The listing builds one solid part. Answer for the finished solid, in the listing's coordinates (mm). Give positions to 0.01 mm unless a question says otherwise; leave off trailing zeros. Order: outer loops, then holes, each group sorted by start corner. A loop starts at its lowest first (then second) coordinate and runs counter-clockwise, first axis right, second up.
```python
from build123d import *

# Parameters (mm, degrees)
SKETCH1_W           = 1155
SKETCH1_H           = 80
BOSS_EXTRUDE1_DEPTH = 12
SKETCH2_R           = 9
CUT_EXTRUDE1_DEPTH  = 580.007987855
LPATTERN1_COUNT     = 4
LPATTERN1_PITCH     = 366
SKETCH3_W           = 60
SKETCH3_H           = 98
SKETCH3_R           = 10
BOSS_EXTRUDE2_DEPTH = 12
SKETCH4_W           = 60
SKETCH4_H           = 12
BOSS_EXTRUDE3_DEPTH = 52.5
SKETCH6_W           = 60
SKETCH6_H           = 110
SKETCH6_R           = 10
BOSS_EXTRUDE4_DEPTH = 12
SKETCH7_W           = 60
SKETCH7_H           = 98
CUT_EXTRUDE2_DEPTH  = 12


with BuildPart() as part:
    # Sketch1 → Boss-Extrude1 (new body)
    with BuildSketch(Plane(origin=(0, 0, 0), x_dir=(1, 0, 0), z_dir=(0, 1, 0))):
        Rectangle(SKETCH1_W, SKETCH1_H)
    extrude(amount=BOSS_EXTRUDE1_DEPTH)

    # Sketch2 → Cut-Extrude1 (cut, symmetric)
    with BuildSketch(Plane(origin=(0, 12, 0), x_dir=(1, 0, 0), z_dir=(0, 1, 0))):
        with Locations(Location((-549, 0, 0), (0, 0, 270))):
            Circle(SKETCH2_R)
    cut_extrude1 = extrude(amount=CUT_EXTRUDE1_DEPTH, both=True, mode=Mode.SUBTRACT)

    # LPattern1: Cut-Extrude1 ×4
    with Locations(*[(i * LPATTERN1_PITCH, 0, 0) for i in range(1, LPATTERN1_COUNT)]):
        add(cut_extrude1, mode=Mode.SUBTRACT)

    # Sketch3 → Boss-Extrude2 (add)
    with BuildSketch(Plane(origin=(0, 12, 0), x_dir=(1, 0, 0), z_dir=(0, 1, 0))):
        with Locations((-427.5, -89)):
            Rectangle(SKETCH3_W, SKETCH3_H)
        with Locations(Location((-427.5, -108, 0), (0, 0, 270))):
            Circle(SKETCH3_R, mode=Mode.SUBTRACT)
    extrude(amount=-BOSS_EXTRUDE2_DEPTH)

    # Sketch4 → Boss-Extrude3 (add)
    with BuildSketch(Plane(origin=(0, 0, 0), x_dir=(-1, 0, 0), z_dir=(0, -1, 0))):
        with Locations((427.5, -34)):
            Rectangle(SKETCH4_W, SKETCH4_H)
    extrude(amount=BOSS_EXTRUDE3_DEPTH)

    # Sketch6 → Boss-Extrude4 (add)
    with BuildSketch(Plane.XZ.offset(52.5)):
        with Locations((-427.5, 83)):
            Rectangle(SKETCH6_W, SKETCH6_H)
        with Locations(Location((-427.5, 108, 0), (0, 0, 90))):
            Circle(SKETCH6_R, mode=Mode.SUBTRACT)
    extrude(amount=BOSS_EXTRUDE4_DEPTH)

    # Sketch7 → Cut-Extrude2 (cut)
    with BuildSketch(Plane(origin=(0, 12, 0), x_dir=(1, 0, 0), z_dir=(0, 1, 0))):
        with Locations((-427.5, -89)):
            Rectangle(SKETCH7_W, SKETCH7_H)
    extrude(amount=-CUT_EXTRUDE2_DEPTH, mode=Mode.SUBTRACT)


solid = part.part
```
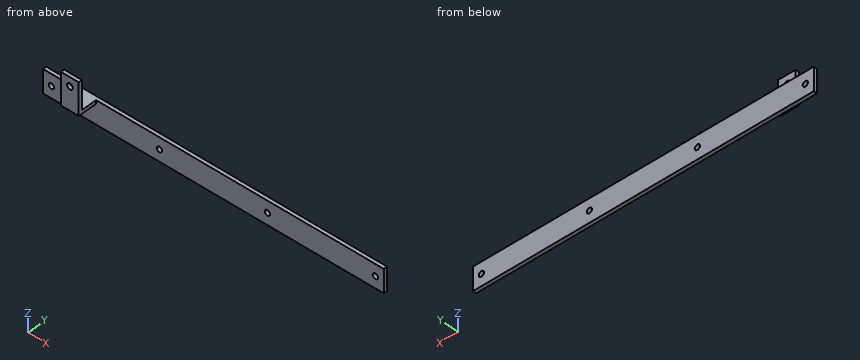
1) Find section C-C (y = -25). Write down the section's boundary in (x, z).
Geometry says:
outline: (-457.5, 28) - (-397.5, 28) - (-397.5, 40) - (-457.5, 40) - close
2) Find section B-B (z = 108). Write down the section's boundary in (x, y), then the cut area to 3 significant figures.
Geometry says:
outline: (-457.5, -64.5) - (-437.5, -64.5) - (-437.5, -52.5) - (-457.5, -52.5) - close; (-417.5, -64.5) - (-397.5, -64.5) - (-397.5, -52.5) - (-417.5, -52.5) - close
area: 480 mm2
3) Find section A-A (x = -427.5). Write down the section's boundary in (y, z), then the cut area to 3 significant figures.
Geometry says:
outline: (-64.5, 28) - (0, 28) - (0, -40) - (12, -40) - (12, 40) - (-52.5, 40) - (-52.5, 98) - (-64.5, 98) - close; (-64.5, 118) - (-52.5, 118) - (-52.5, 138) - (-64.5, 138) - close
area: 2,670 mm2
4) Find section D-D (x = -137). Write down the section's boundary in (y, z), then the cut area to 3 significant figures.
Geometry says:
outline: (0, -40) - (12, -40) - (12, 40) - (0, 40) - close
area: 960 mm2
5) Given P1, Ø6, axis at x = -399, y = -7.5, coming from the +Z side; P2, Ø10, axis at x = 202.5, z = 40, coming from the -Y side, each flat-ended and moving along its own axis, determine where each tip first touches the part or whether it passes through.
Geometry says:
P1: stops at z = 40
P2: stops at y = 0
6) Straight lines are drawn through the part: probe 1 along X at (y, z) = (7.75, 0); probe 2 along Z at (x, y) = (549, 5.25); probe 3 along X at (y, z) = (-60.75, 108). For each, find the intervals that lie inside material, in ascending order.
Geometry says:
probe 1: x = -577.5 to -558, -540 to -192, -174 to 174, 192 to 540, 558 to 577.5
probe 2: z = -40 to -9, 9 to 40
probe 3: x = -457.5 to -437.5, -417.5 to -397.5
